The figure shows three views and two pictorial views of one solid part (mm, origin at its lowest corner). Answer the questions. Round coordinates to 2 decimals unless told otherwise and drop trailing zeros. Write each loop counter-clockwise with the first axis right and the second up, starting at its lowest first coordinate (ties: lowest second). Pieces come first, ordered by that corner, then holes.
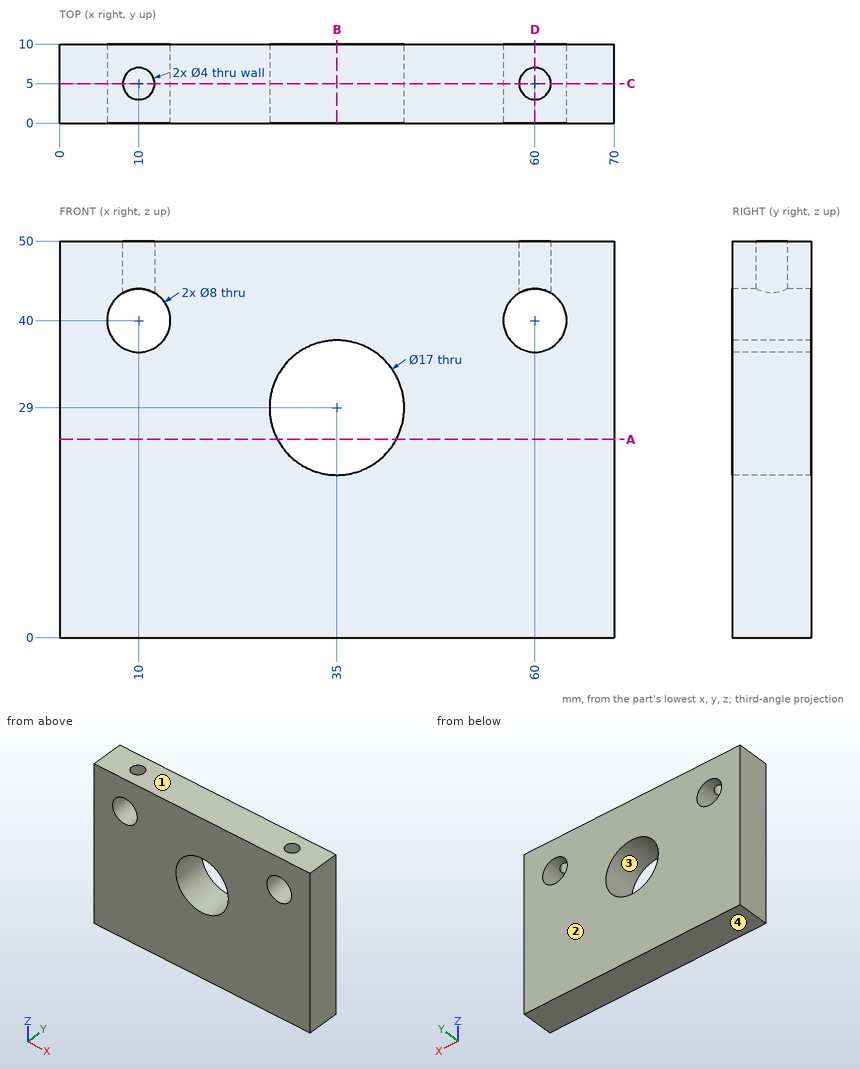
Q1. Section C-C (y = 5) is taken. Determine the outline of the cut face in (x, z), then the cut area to 3 significant figures.
Verdict:
outline: (0, 0) - (70, 0) - (70, 50) - (62, 50) - (62, 43.46) arc R4 cw (long way) to (58, 43.46) - (58, 50) - (12, 50) - (12, 43.46) arc R4 cw (long way) to (8, 43.46) - (8, 50) - (0, 50) - close; hole circle Ø17 at (35, 29)
area: 3,120 mm2
Q2. Section D-D (x = 60) is taken. Determine the outline of the cut face in (y, z), then the cut area to 3 significant figures.
Verdict:
outline: (0, 0) - (10, 0) - (10, 36) - (0, 36) - close; (0, 44) - (3, 44) - (3, 50) - (0, 50) - close; (7, 44) - (10, 44) - (10, 50) - (7, 50) - close
area: 396 mm2
Q3. Section A-A (z = 25) is taken. Determine the outline of the cut face in (x, y), then the cut area to 3 significant figures.
Verdict:
outline: (0, 0) - (27.5, 0) - (27.5, 10) - (0, 10) - close; (42.5, 0) - (70, 0) - (70, 10) - (42.5, 10) - close
area: 550 mm2
Q4. Section B-B (x = 35) is taken. Determine the outline of the cut face in (y, z).
Verdict:
outline: (0, 0) - (10, 0) - (10, 20.5) - (0, 20.5) - close; (0, 37.5) - (10, 37.5) - (10, 50) - (0, 50) - close
Q5. Determine the mould class of the marked faces 1, 2, 3 and 4 for opening direction Z: pulls with the +Z half, pulls with the -Z half, needs draft (parallel to the pull), parting line crosses it, or undercut.
Verdict:
face 1: pulls with the +Z half
face 2: needs draft
face 3: undercut
face 4: pulls with the -Z half
Q6. Straight lines are drawn through the part: probe 1 along Z at (x, y) = (35, 7.5); probe 2 along Z at (x, y) = (60, 9); probe 3 along Y at (x, z) = (10, 48.5). For each, find the intervals that lie inside material, in ascending order.
Verdict:
probe 1: z = 0 to 20.5, 37.5 to 50
probe 2: z = 0 to 36, 44 to 50
probe 3: y = 0 to 3, 7 to 10
